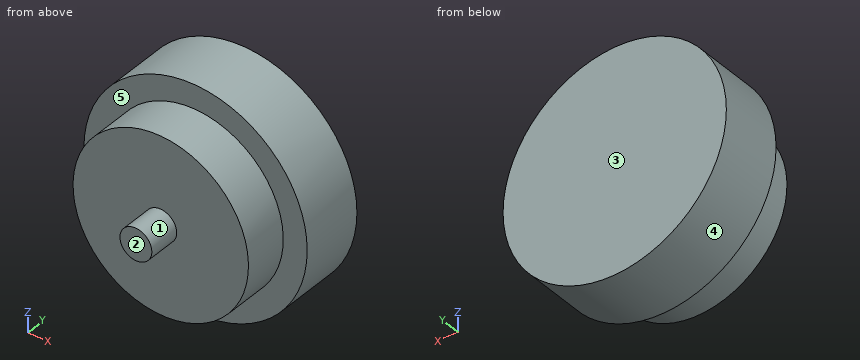
```python
from build123d import *

# Parameters (mm, degrees)
SKETCH1_R           = 1.25
BOSS_EXTRUDE1_DEPTH = 2.5
SKETCH2_R           = 6.875
BOSS_EXTRUDE2_DEPTH = 3.5
SKETCH3_R           = 8.75
BOSS_EXTRUDE3_DEPTH = 5


with BuildPart() as part:
    # Sketch1 → Boss-Extrude1 (new body)
    with BuildSketch(Plane(origin=(0, 0, 0), x_dir=(1, 0, 0), z_dir=(0, 1, 0))):
        with Locations(Location((0, 0, 0), (0, 0, 270))):
            Circle(SKETCH1_R)
    extrude(amount=BOSS_EXTRUDE1_DEPTH)

    # Sketch2 → Boss-Extrude2 (add)
    with BuildSketch(Plane(origin=(0, 2.5, 0), x_dir=(1, 0, 0), z_dir=(0, 1, 0))):
        with Locations(Location((0, 0, 0), (0, 0, 270))):
            Circle(SKETCH2_R)
    extrude(amount=BOSS_EXTRUDE2_DEPTH)

    # Sketch3 → Boss-Extrude3 (add)
    with BuildSketch(Plane(origin=(0, 6, 0), x_dir=(1, 0, 0), z_dir=(0, 1, 0))):
        with Locations(Location((0, 0, 0), (0, 0, 270))):
            Circle(SKETCH3_R)
    extrude(amount=BOSS_EXTRUDE3_DEPTH)


solid = part.part
```
Verification items for the finished model (mm, model axes). Face numbers are marked on the shaded views. A direction names the side the tool comes from. Give positions to 0.01 mm unless a question says otherwise; leave off trailing zeros. Order: outer loops, then holes, each group sorted by start corner. A loop starts at its lowest first (then second) coordinate and runs counter-clockwise, first axis right, second up. Notation, with made-up numbers: M 32.5,80.25 L 41.5,80.25 A15 ccw 41.5,94.25 Z; hole C 75.25,-11.5 d3. An arc over 180 degrees is marked long. Answer in a Markdown table with one row per item. Add a question column.
Item 1: Section check C-C, the plane y = 4.25. Enter the section's corners in (x, z) (3 decimals), and give its area (3 significant figures).
Item 2: Gauge pin test, flat ends, axial feed: pin 1 (1.5 mm diameter, centred on x = 4, y = 3, fed in from -Z); pin 2 (2 mm diameter, centred on x = 3.5, y = 2, fed in from -Z); pin 3 (5 mm diameter, centred on x = 6, z = 5, fed in from -Y). Record the tip position at first contact, or that the pin passes through.
Item 3: Section check D-D, the plane x = 3.75. Enter the section's corners in (y, z), and give its area (3 significant figures).
Item 4: Section check A-A, the plane z = 0. Enter the section's corners in (x, y) (3 decimals).
Item 5: Scan lines: probe 1 along Y at (x, z) = (4, -4); probe 2 along Y at (x, z) = (-6.25, -6); probe 3 along X at (y, z) = (7, 6). Record each from-to range of solid material in increasing order. Write a range as from..to.
Item 6: Mould release check, pull along Y, two halves, no side actions. Record for the marked faces 1, 2 and 3: released by +Y, released by -Y, zero draft, split by the parting line, or undercut.
Item 7: Tool access check on the marked faces 4 and 5. Record the directions out of +Z, -Z, +X, -X, +Y, -Y that give a thin tool (end or side, any length) a straight path to the whole face; none if there is none.
Item 8: Section check B-B, the plane x = 0. Enter the section's corners in (y, z) (3 decimals).
Filled sheet:
| question | item | result |
|---|---|---|
| 1 | outline | C 0,0 d13.75 |
| 1 | area | 148 mm^2 |
| 2 | pin 1 | stops at z = -6.06 |
| 2 | pin 2 | stops at z = -6.35 |
| 2 | pin 3 | stops at y = 2.5 |
| 3 | outline | M 2.5,-5.76 L 6,-5.76 L 6,-7.91 L 11,-7.91 L 11,7.91 L 6,7.91 L 6,5.76 L 2.5,5.76 Z |
| 3 | area | 119 mm^2 |
| 4 | outline | M -8.75,6 L -6.875,6 L -6.875,2.5 L -1.25,2.5 L -1.25,0 L 1.25,0 L 1.25,2.5 L 6.875,2.5 L 6.875,6 L 8.75,6 L 8.75,11 L -8.75,11 Z |
| 5 | probe 1 | y = 2.5..11 |
| 5 | probe 2 | y = 6..11 |
| 5 | probe 3 | x = -6.37..6.37 |
| 6 | face 1 | zero draft |
| 6 | face 2 | released by -Y |
| 6 | face 3 | released by +Y |
| 7 | face 4 | +Y, -Y |
| 7 | face 5 | -Y |
| 8 | outline | M 0,-1.25 L 2.5,-1.25 L 2.5,-6.875 L 6,-6.875 L 6,-8.75 L 11,-8.75 L 11,8.75 L 6,8.75 L 6,6.875 L 2.5,6.875 L 2.5,1.25 L 0,1.25 Z |
